Verification items for the finished model (mm, model axes). A direction names the side the tool comes from. Give positions to 0.01 mm unless a question says otherwise; leave off trailing zeros. Loops run counter-clockwise (first coordinate to the right, second up) from the corner with the lowest first, then second, coordinate; pieces in that order, holes last. Notation, with made-up numbers: (73, -19) - (132, -19) arc R7 cw to (132, -9) - close; hole circle Ø1 at (-32, -14). An arc over 180 degrees is marked (long way). Answer in a Markdown table with one row per item.
Autodesk Inventor part; units mm, degrees
ref_plane "YZ Plane" through (0, 0, 0) normal (1, 0, 0) x (0, 1, 0)
ref_plane "XZ Plane" through (0, 0, 0) normal (0, 1, 0) x (-1, 0, 0)
ref_plane "XY Plane" through (0, 0, 0) normal (0, 0, 1) x (1, 0, 0)
sketch "スケッチ1" plane through (0, 0, 0) normal (1, 0, 0) x (0, 1, 0)
  line L0 (30, 15) -> (120, 15)
  line L1 (120, 15) -> (120, -15)
  line L2 (120, -15) -> (30, -15)
  line L3 (0, -15) -> (0, 15)
  line L4 (30, 100) -> (0, 100)
  line L5 (0, 100) -> (0, -100)
  line L6 (0, -100) -> (30, -100)
  line L7 (30, -100) -> (30, -15)
  line L8 (30, 15) -> (30, 100)
  point P0 (0, 0)
  point P1 (0, 0)
  dimension "d0" = 30
  dimension "d1" = 120
  dimension "d2" = 30
  dimension "d3" = 200
extrude "押し出し1" add sketch "スケッチ1" along normal blind 30
sketch "スケッチ2" plane through (30, 0, 0) normal (1, 0, 0) x (0, 0, -1)
  line L0 (-23.0571, 9) -> (23.0571, 9)
  line L1 (5.5, 20) -> (5.5, 105)
  line L2 (5.5, 105) -> (-5.5, 105)
  line L3 (-5.5, 105) -> (-5.5, 20)
  line L4 (-100, 0) -> (100, 0)
  line L5 (-85, 9) -> (85, 9)
  line L6 (85, 9) -> (85, 20)
  line L7 (-85, 20) -> (-85, 9)
  line L8 (85, 20) -> (5.5, 20)
  line L9 (-5.5, 20) -> (-85, 20)
  point P0 (0, 0)
  point P1 (0, 9)
  dimension "d6" = 11
  dimension "d8" = 11
  dimension "d9" = 170
  dimension "d10" = 9
  dimension "d11" = 11
  dimension "d12" = 85
sketch "スケッチ3" plane through (30, 0, 0) normal (1, 0, 0) x (0, 0, -1)
  point P0 (0, 0)
extrude "押し出し2" cut sketch "スケッチ2" against normal blind 10
fillet "フィレット1" radius 3 1 edges at (15, 30, 100)
fillet "フィレット2" radius 3 1 edges at (15, 0, 100)
fillet "フィレット3" radius 3 1 edges at (15, 0, -100)
fillet "フィレット4" radius 3 1 edges at (15, 30, -100)
fillet "フィレット5" radius 3 1 edges at (25, 20, -85)
fillet "フィレット6" radius 3 1 edges at (25, 9, -85)
fillet "フィレット7" radius 3 1 edges at (25, 9, 85)
fillet "フィレット8" radius 3 1 edges at (25, 20, 85)
fillet "フィレット9" radius 3 1 edges at (25, 105, 5.5)
fillet "フィレット10" radius 3 1 edges at (25, 105, -5.5)
fillet "フィレット11" radius 3 1 edges at (15, 30, 15)
fillet "フィレット12" radius 3 1 edges at (15, 30, -15)
equation "\"d11\" = d8"
properties part number "Main"
Q1. Sectioned sample at B-B (x = 23). Record the cut outline in (y, z), and give its area (3 significant figures).
Completed:
| item | result |
|---|---|
| outline | (0, -97) arc R3 ccw to (3, -100) - (27, -100) arc R3 ccw to (30, -97) - (30, -18) arc R3 cw to (33, -15) - (120, -15) - (120, 15) - (33, 15) arc R3 cw to (30, 18) - (30, 97) arc R3 ccw to (27, 100) - (3, 100) arc R3 ccw to (0, 97) - close; hole (9, -82) arc R3 ccw to (12, -85) - (17, -85) arc R3 ccw to (20, -82) - (20, -5.5) - (102, -5.5) arc R3 ccw to (105, -2.5) - (105, 2.5) arc R3 ccw to (102, 5.5) - (20, 5.5) - (20, 82) arc R3 ccw to (17, 85) - (12, 85) arc R3 ccw to (9, 82) - close |
| area | 5,900 mm^2 |
Q2. Tool access check on faces 1 (the face through (0, 29, -7)), 2 (the face through (15, 77, -15)), 3 (the face through (15, 15, 100)), 4 (the face through (25, 62, 5.5)), 5 (the face through (15, 76, 15)). Record the directions out of +Z, -Z, +X, -X, +Y, -Y that give a thin tool (end or side, any length) a straight path to the whole face; none if there is none.
Completed:
| item | result |
|---|---|
| face 1 | +Z, -Z, -X, +Y, -Y |
| face 2 | -Z, +X, -X, +Y |
| face 3 | +Z, +X, -X, +Y, -Y |
| face 4 | +X |
| face 5 | +Z, +X, -X, +Y |
Q3. Go/stop test with flat-tipped pins: P1, Ø1, axis at x = 26, z = -55, coming from the +Y side; P2, Ø15, axis at x = 20, y = 93, coming from the -Z side; P3, Ø5, axis at x = 23.5, y = 46.5, coming from the +Z side. Record where each tip stops, or that it passes through.
Completed:
| item | result |
|---|---|
| P1 | y = 30 |
| P2 | z = -15 |
| P3 | z = 15 |
Q4. Sectioned sample at D-D (x = 5). Record the cut outline in (y, z), and give its area (3 significant figures).
Completed:
| item | result |
|---|---|
| outline | (0, -97) arc R3 ccw to (3, -100) - (27, -100) arc R3 ccw to (30, -97) - (30, -18) arc R3 cw to (33, -15) - (120, -15) - (120, 15) - (33, 15) arc R3 cw to (30, 18) - (30, 97) arc R3 ccw to (27, 100) - (3, 100) arc R3 ccw to (0, 97) - close |
| area | 8,700 mm^2 |
Q5. Sectioned sample at A-A (y = 24.5). Record the cut outline in (x, z).
Completed:
| item | result |
|---|---|
| outline | (0, -100) - (30, -100) - (30, -5.5) - (20, -5.5) - (20, 5.5) - (30, 5.5) - (30, 100) - (0, 100) - close |
Q6. Thickness scan on line 1 (Y direction, x = 21, z = -75); line 2 (Z direction, x = 20.5, y = 67); line 3 (Y direction, x = 2, z = 91.5). Record the ranges inside material, lowest first.
Completed:
| item | result |
|---|---|
| line 1 | 0 to 9, 20 to 30 |
| line 2 | -15 to -5.5, 5.5 to 15 |
| line 3 | 0 to 30 |
Q7. Sectioned sample at C-C (z = 21.5). Record the cut outline in (x, y).
Completed:
| item | result |
|---|---|
| outline | (0, 0) - (30, 0) - (30, 9) - (20, 9) - (20, 20) - (30, 20) - (30, 30) - (0, 30) - close |
